Work out the finished part from the listing and answer in its coordinate system (mm). Face numbers are marked on the shaded views. A direction names the side the tool comes from. Round coordinates to 2 decimals unless told otherwise and drop trailing zeros. Order: outer loops, then holes, each group sorted by start corner. A loop starts at its lowest first (then second) coordinate and runs counter-clockwise, first axis right, second up. Notation, with made-up numbers: (-20.5, 52.5) - (1.5, 52.5) arc R33 ccw to (1.5, 88.5) - close; hole circle Ø1 at (29, -27.5). An arc over 180 degrees is marked (long way). Use CSV: the item, a comma, the result in double quotes.
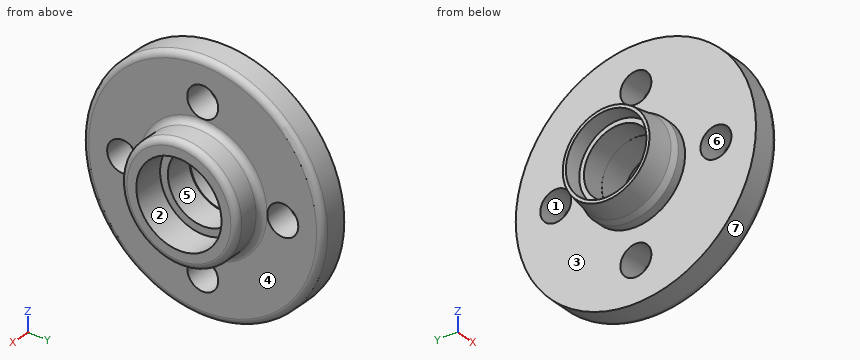
from build123d import *

# Parameters (mm, degrees)
F0_R     = 77.5
F0_R_2   = 22.5
F1_DEPTH = 18
F2_R     = 37.5
F2_R_2   = 27.5
F3_DEPTH = 20
F4_R     = 4
F7_R     = 10
F8_DEPTH = 25


with BuildPart() as f1:
    # F0 (on Right) → F1 (new body)
    with BuildSketch(Plane.YZ):
        Circle(F0_R)
        Circle(F0_R_2, mode=Mode.SUBTRACT)
    extrude(amount=F1_DEPTH)

    # F2 (on face) → F3 (join)
    with BuildSketch(Plane.YZ.offset(18)):
        Circle(F2_R)
        Circle(F2_R_2, mode=Mode.SUBTRACT)
    extrude(amount=F3_DEPTH)

    # F4
    f4_edges = [f1.edges().sort_by_distance(p)[0] for p in [
        (28, 37.5, 0),
        (18, -37.5, 0),
        (38, -37.5, 0),
        (18, -77.5, 0),
    ]]
    fillet(f4_edges, radius=F4_R)

    # F5 (on Front) → F6 (revolve)
    with BuildSketch(Plane.XZ):
        Polygon((-5.721824, -31.75), (0, -31.75), (0, -22), (-15, -22), (-15, -25), (-25, -26), (-25, -28), (-10, -30.354747), align=None)
    revolve(axis=Axis((-7.5, 0, 0), (-1, 0, 0)))

    # F7 (on Right) → F8 (cut)
    with BuildSketch(Plane.YZ):
        with Locations((0, 51.6636)):
            Circle(F7_R)
        with Locations((-51.6636, 0)):
            Circle(F7_R)
        with Locations((0, -51.6636)):
            Circle(F7_R)
        with Locations((51.6636, 0)):
            Circle(F7_R)
    extrude(amount=F8_DEPTH, mode=Mode.SUBTRACT)


solid = f1.part
(1) Find section A-A (y = 0). State how many separate pieces and enclosed holes the cut face has, and give its area (3 significant figures).
Findings below:
separate pieces,"4"
enclosed holes,"0"
area,"1,990 mm²"
(2) Find the intervals of material crossed by L1, parallel to Z at x = 12.25, y = 0; L2, parallel to Y at x = -10, z = 0; L3, parallel to X at y = -53.5, z = 16, in increasing order. Write a range as from..to.
Findings below:
L1,"z = -77.5..-61.66, -41.66..-22.5, 22.5..41.66, 61.66..77.5"
L2,"y = -30.35..-22, 22..30.35"
L3,"x = 0..18"
(3) Each of these flat-tipped pins is pushed along its axis until it touches: pin 1 (3 mm diameter, centred on x = 16, z = 43.5, fed in from +Y); pin 2 (12 mm diameter, centred on y = 0, z = -51.66, fed in from -X); pin 3 (5 mm diameter, centred on y = 19.5, z = 32, fed in from -X); pin 4 (23 mm diameter, centred on y = 51.66, z = 0, fed in from +X). Where does it stop, or does it pass through?
Findings below:
pin 1,"stops at y = 64.76"
pin 2,"passes through"
pin 3,"stops at x = 0"
pin 4,"stops at x = 18.23"
(4) The mould has two halves that part along Y. Classify the marked faces 4, 5, 6 and 7: released by +Y, released by -Y, zero draft, split by the parting line, or undercut.
Findings below:
face 4,"zero draft"
face 5,"undercut"
face 6,"undercut"
face 7,"split by the parting line"
(5) Find section B-B (x = 3.5). Determine the outline of the cut face in (y, z), and give its area (3 significant figures).
Findings below:
outline,"circle Ø155 at (0, 0); hole circle Ø20 at (-51.66, 0); hole circle Ø45 at (0, 0); hole circle Ø20 at (0, -51.66); hole circle Ø20 at (0, 51.66); hole circle Ø20 at (51.66, 0)"
area,"16,000 mm²"
(6) For the marked faces 1, 2 and 3, determine the directions among +Z, -Z, +X, -X, +Y, -Y from which every point of the face is accessible in a straight line to the end or side of a thin tool.
Findings below:
face 1,"+X, -X"
face 2,"+X"
face 3,"-X"
